Input: part model. Units: mm. Frame: model coordinates. A direction names the side the tool comes from. Give positions to 0.01 mm unless a question says otherwise; leave off trailing zeros. Write each loop counter-clockwise with the first axis right and the second up, starting at its lowest first coordinate (ties: lowest second). Pieces come first, ordered by that corner, then holes. Notation, with made-up numbers: (23, -4.5) -> (37, -4.5) arc R29 cw to (37, 34.5) -> close; hole circle Ø9 at (48, 68.25). An arc over 180 degrees is marked (long way). Return JSON: item names as keys, results as strings. Group by question number.
Item 1: Pin query (flat end, axial travel): P1, Ø10, axis at y = 10.5, z = -26, coming from the -X side; P2, Ø2, axis at y = 33, z = -19.5, coming from the +X side; P3, Ø6, axis at x = -18.5, z = -20, coming from the +Y side; P4, Ø3, axis at x = 11, z = 30, coming from the +Y side. Return the tip coordinate at first contact, or that it passes through.
Item 2: Set-up query: faces 1 (the face through (17.8, 49.5, 0.5)), 2 (the face through (21.375, 20.557, 0.56)). Return all of +Z, -Z, +X, -X, +Y, -Y with unobstructed straight access to the full face (end or side cutting, diameter ignored); none if empty.
Item 3: Mould query, pull axis X, two halves, no side actions, for faces 3 (the face through (11.601, -1.521, -31.908)), 4 (the face through (-23, -1, -37)), 5 (the face through (-1, 0, -1)). Classes: released by +X, released by -X, zero draft, split by the parting line, or undercut.
Item 4: Line query: line 1 (Y direction, x = 15, z = 15.5); line 2 (X direction, y = -1, z = 0); line 3 (X direction, y = 4, z = -10). Output: solid intervals per line, ascending. Write a range as [from, to].
Item 5: Section B-B, the plane z = -30. Return loops of the section in (x, y), then the cut area to 3 significant figures.
Item 6: Section D-D, the plane z = -16. Return loops of the section in (x, y), then the cut area to 3 significant figures.
Item 7: Section C-C, the plane x = 11. Return loops of the section in (y, z).
Item 8: Section A-A, the plane x = -19. Return loops of the section in (y, z).
from build123d import *

# Parameters (mm, degrees)
SKETCH1_W                    = 50
SKETCH1_H                    = 80
BASE_FLANGE1_DEPTH           = 3
EDGE_FLANGE1_STRIP_CUT_DEPTH = 80
EDGE_FLANGE1_DEPTH           = 80
CHAMFER1_SIZE                = 5
SKETCH7_R                    = 5.25
CUT_EXTRUDE1_DEPTH           = 10
CUT_EXTRUDE2_REACH           = 73.776
SKETCH8_R                    = 2


# Sheet-metal steps are written as plain solids
with BuildPart() as part:
    # Sketch1 → Base-Flange1 (new body)
    with BuildSketch(Plane(origin=(0, 0, 0), x_dir=(1, 0, 0), z_dir=(0, 1, 0))):
        Rectangle(SKETCH1_W, SKETCH1_H)
    extrude(amount=-BASE_FLANGE1_DEPTH)

    # Edge-Flange1 strip (across the edge) → Edge-Flange1 strip cut (cut)
    with BuildSketch(Plane(origin=(25, 0, 40), x_dir=(-0.9848077530122087, -0.17364817766692717, 0), z_dir=(0, 0, -1))):
        Polygon((-15.323305866, -5.748192093), (2.2814168, -2.6440045), (1.760472267, 0.310418759), (-15.844250399, -2.793768834), align=None)
    extrude(amount=EDGE_FLANGE1_STRIP_CUT_DEPTH, mode=Mode.SUBTRACT)

    # Edge-Flange1 section (across the edge) → Edge-Flange1 (add)
    with BuildSketch(Plane(origin=(25, 0, 40), x_dir=(-0.9848077530122087, -0.17364817766692717, 0), z_dir=(0, 0, -1))):
        with BuildLine():
            Line((-3, 1.787630389), (-3, 50))
            Line((-3, 50), (0, 50))
            Line((0, 50), (0, 1.787630389))
            ThreePointArc((0, 1.787630389), (0.535818585, 0.638563724), (1.760472267, 0.310418759))
            Line((1.760472267, 0.310418759), (2.2814168, -2.6440045))
            ThreePointArc((2.2814168, -2.6440045), (-1.392544244, -1.659569605), (-3, 1.787630389))
        make_face()
    extrude(amount=EDGE_FLANGE1_DEPTH)

    # Chamfer1
    chamfer1_edges = [part.edges().sort_by_distance(p)[0] for p in [
        (17.794802746, 49.500859917, 40),
        (17.794802746, 49.500859917, -40),
        (-25, -1.5, 40),
        (-25, -1.5, -40),
    ]]
    chamfer(chamfer1_edges, length=CHAMFER1_SIZE)

    # Sketch7 → Cut-Extrude1 (cut)
    with BuildSketch(Plane(origin=(27.200581019, 4.796196325, 0), x_dir=(0, 0, -1), z_dir=(0.9848077530122087, 0.1736481776669272, 0))):
        with Locations(Location((0, 22.158795558, 0), (0, 0, 90))):
            Circle(SKETCH7_R)
    extrude(amount=-CUT_EXTRUDE1_DEPTH, mode=Mode.SUBTRACT)

    # Sketch8 → Cut-Extrude2 (cut, up to next)
    with BuildSketch(Plane.XZ.offset(3), mode=Mode.PRIVATE) as cut_extrude2_sk1:
        with Locations(Location((-19, 0, 0), (0, 0, 270))):
            Circle(SKETCH8_R)
    cut_extrude2_tool1 = extrude(cut_extrude2_sk1.sketch, amount=-CUT_EXTRUDE2_REACH, mode=Mode.PRIVATE) & part.part
    # Sketch8 → Cut-Extrude2 (cut, up to next)
    with BuildSketch(Plane.XZ.offset(3), mode=Mode.PRIVATE) as cut_extrude2_sk2:
        with Locations(Location((11, 30, 0), (0, 0, 270))):
            Circle(SKETCH8_R)
    cut_extrude2_tool2 = extrude(cut_extrude2_sk2.sketch, amount=-CUT_EXTRUDE2_REACH, mode=Mode.PRIVATE) & part.part
    # Sketch8 → Cut-Extrude2 (cut, up to next)
    with BuildSketch(Plane.XZ.offset(3), mode=Mode.PRIVATE) as cut_extrude2_sk3:
        with Locations(Location((11, -30, 0), (0, 0, 270))):
            Circle(SKETCH8_R)
    cut_extrude2_tool3 = extrude(cut_extrude2_sk3.sketch, amount=-CUT_EXTRUDE2_REACH, mode=Mode.PRIVATE) & part.part
    add(cut_extrude2_tool1.solids().sort_by_distance((-19, -3, 0))[0], mode=Mode.SUBTRACT)
    add(cut_extrude2_tool2.solids().sort_by_distance((11, -3, 30))[0], mode=Mode.SUBTRACT)
    add(cut_extrude2_tool3.solids().sort_by_distance((11, -3, -30))[0], mode=Mode.SUBTRACT)


solid = part.part
Answer below:
{
 "1": {"P1": "stops at x = 22.27", "P2": "stops at x = 22.4", "P3": "stops at y = 0", "P4": "passes through"},
 "2": {"face 1": "+Z, -Z, -X, +Y", "face 2": "+Z, -Z, -X"},
 "3": {"face 3": "undercut", "face 4": "released by -X", "face 5": "zero draft"},
 "4": {"line 1": "y = [-3, 0]", "line 2": "x = [-25, -21], [-17, 26.95]", "line 3": "x = [24.29, 27.34]"},
 "5": {"outline": "(-25, -3) -> (9, -3) -> (9, 0) -> (-25, 0) -> close; (13, -3) -> (23.21, -3) arc R4.5 ccw to (27.64, 2.28) -> (19.27, 49.76) -> (16.32, 49.24) -> (24.69, 1.76) arc R1.5 cw to (23.21, 0) -> (13, 0) -> close", "area": "293 mm2"},
 "6": {"outline": "(-25, -3) -> (23.21, -3) arc R4.5 ccw to (27.64, 2.28) -> (19.27, 49.76) -> (16.32, 49.24) -> (24.69, 1.76) arc R1.5 cw to (23.21, 0) -> (-25, 0) -> close", "area": "305 mm2"},
 "7": {"outline": "(-3, -40) -> (0, -40) -> (0, -32) -> (-3, -32) -> close; (-3, -28) -> (0, -28) -> (0, 28) -> (-3, 28) -> close; (-3, 32) -> (0, 32) -> (0, 40) -> (-3, 40) -> close"},
 "8": {"outline": "(-3, -40) -> (0, -40) -> (0, -2) -> (-3, -2) -> close; (-3, 2) -> (0, 2) -> (0, 40) -> (-3, 40) -> close"}
}
